Geometry check sheet. Reference: the model listing, model coordinates, mm. A direction names the side the tool comes from. Coordinates: 2 decimals unless noted, no trailing zeros. Order: outer loops, then holes, each group sorted by start corner. A loop starts at its lowest first (then second) coordinate and runs counter-clockwise, first axis right, second up. Notation, with made-up numbers: M -35.75,61.25 L -16.75,61.25 A34 ccw -16.75,99.25 Z; hole C 24.25,-9.5 d7. An arc over 180 degrees is marked long. One line per item, written item: value. Start each with the question number.
1) Sectioned sample at B-B, the plane x = -39. Enter the section's corners in (y, z).
2) Thickness scan on L1, parallel to X at y = -33, z = 1.3; L2, parallel to Y at x = -44, z = -0.3; L3, parallel to Y at x = -35, z = 0.65. Record the ranges inside material, lowest first. Write a range as from..to.
3) Draft check along X on faces 1 (the flat face through (-9, -11, 1.5)), 2 (the flat face through (-10, -27, 0)), 3 (the flat face through (0, 0, 0.5)). Enter one of: pulls with the +X half, pulls with the -X half, needs draft (parallel to the pull), parting line crosses it, or undercut.
4) Go/stop test with flat-tipped pins: P1, Ø1.5, axis at y = -33, z = -0.5, coming from the -X side; P2, Ø2.5, axis at x = -1, y = -0.5, coming from the -Z side; P3, Ø1.5, axis at y = -18.5, z = 0.5, coming from the +X side. Record where each tip stops, or that it passes through.
5) Access from +Z, -Z, +X, -X, +Y, -Y to the whole of each face (thin tool, end or side, straight path). Record for faces 4 (the cylindrical face through (-10.365, -49.663, 0.021)), 5 (the cylindrical face through (-30.09, -0.74, 0.02)), 6 (the cylindrical face through (0.54, -2.44, -0.51)).
6) Sectioned sample at A-A, the plane y = -9.5. Enter the section's corners in (x, z), then the cut area to 3 significant figures.
```python
from build123d import *

# Parameters (mm, degrees)
BOSS_EXTRU_1_DEPTH      = 1.5
BOSS_EXTRU_2_DEPTH      = 3
ESQUISSE2_R             = 2.5
ENL_V_MAT_EXTRU_3_DEPTH = 2
CONG_1_R                = 10


with BuildPart() as part:
    # Esquisse1 → Boss.-Extru.1 (new body, symmetric)
    with BuildSketch(Plane.XY):
        with BuildLine():
            Line((-10, -45), (-10, -8.660254038))
            ThreePointArc((-10, -8.660254038), (-7.990381057, -1.160254038), (-2.5, 4.330127019))
            ThreePointArc((-2.5, 4.330127019), (4.330127019, 2.5), (2.5, -4.330127019))
            ThreePointArc((2.5, -4.330127019), (0.669872981, -6.160254038), (0, -8.660254038))
            Line((0, -8.660254038), (0, -45))
            ThreePointArc((0, -45), (-0.472828873, -51.132107527), (-1.880137136, -57.11924318))
            ThreePointArc((-1.880137136, -57.11924318), (-8.160025392, -60.369320641), (-11.410102852, -54.089432385))
            ThreePointArc((-11.410102852, -54.089432385), (-10.354621655, -49.599080646), (-10, -45))
        make_face()
    extrude(amount=BOSS_EXTRU_1_DEPTH, both=True)

    # Esquisse4 → Boss.-Extru.2 (add)
    with BuildSketch(Plane.XY.offset(1.5)):
        with BuildLine():
            ThreePointArc((-38.042287627, -6.912622664), (-45.092258789, -7.458430888), (-45.638067013, -0.408459726))
            ThreePointArc((-45.638067013, -0.408459726), (-22.103290159, 11.693784424), (3.175473194, 3.862171668))
            ThreePointArc((3.175473194, 3.862171668), (3.862171668, -3.175473194), (-3.175473194, -3.862171668))
            ThreePointArc((-3.175473194, -3.862171668), (-21.231732732, 1.731837443), (-38.042287627, -6.912622664))
        make_face()
    extrude(amount=-BOSS_EXTRU_2_DEPTH)

    # Esquisse2 → Enlèv. mat.-Extru.3 (cut)
    with BuildSketch(Plane(origin=(0, 0, -1.5), x_dir=(-1, 0, 0), z_dir=(0, 0, -1))):
        Circle(ESQUISSE2_R)
    extrude(amount=-ENL_V_MAT_EXTRU_3_DEPTH, mode=Mode.SUBTRACT)

    # Congé1
    cong_1_edges = [part.edges().sort_by_distance(p)[0] for p in [
        (-7.8041925, -0.846634236, 0),
    ]]
    fillet(cong_1_edges, radius=CONG_1_R)


solid = part.part
```
Final values:
1. outline: M -7.78,-1.5 L 5.59,-1.5 L 5.59,1.5 L -7.78,1.5 Z
2. L1: x = -10..0
2. L2: y = -8.17..1.38
2. L3: y = -3.92..7.98
3. face 1: needs draft
3. face 2: pulls with the -X half
3. face 3: undercut
4. P1: stops at x = -10
4. P2: stops at z = 0.5
4. P3: stops at x = 0
5. face 4: +Z, -Z, -X
5. face 5: +Z, -Z, -Y
5. face 6: -Z
6. outline: M -10,-1.5 L 0,-1.5 L 0,1.5 L -10,1.5 Z
6. area: 30.0 mm^2
